Part model, mm, in its own coordinate system. A direction names the side the tool comes from. Round coordinates to 2 decimals unless told otherwise and drop trailing zeros. Write each loop counter-clockwise with the first axis right and the second up, starting at its lowest first coordinate (ties: lowest second). Pieces come first, ordered by that corner, then holes. Notation, with made-up numbers: M 1,30 L 37,30 A32 cw 37,66 Z; hole C 1.25,87 d5. An arc over 180 degrees is marked long. Use a Markdown table: item, result. Add a question column.
1) Slice it at D-D on z = 1.15. Write the cut outline in (x, y).
2) Slice it at C-C on y = 0. Write the cut outline in (x, z), plus the area to 4 significant figures.
3) Slice it at B-B on x = 0. Write the cut outline in (y, z), plus the area to 3 significant figures.
4) Wall check: probe 1 along Z at (x, y) = (1.65, -3.25); probe 2 along Y at (x, z) = (0.9, 0.3); probe 3 along Z at (x, y) = (0.15, -3.75). Give the ranges that are in metal, low to high.
5) Slice it at A-A on y = -4. Write the cut outline in (x, z), plus the area to 3 significant figures.
6) Which spindle directions (+Z, -Z, +X, -X, +Y, -Y) get a long thin tool onto all of the face, cutting with end or side? Do faces 1 (the face through (0.27, -1.22, -1.13)), 2 (the face through (0, 2.25, 1)). Say none if no direction does.
7) Drop flat-ended pins along their axis: P1, Ø0.7, axis at x = 0, y = -3, coming from the +Z side; P2, Ø2, axis at x = 0.5, z = 0.5, coming from the -Y side; P3, Ø0.7, axis at x = -1.5, y = -3.5, coming from the +Z side; P4, Ø0.7, axis at x = -1.5, y = -4, coming from the -Z side. Give the stop position or say it passes through.
```python
from build123d import *

# Parameters (mm, degrees)
SKETCH_1_W      = 4.5
SKETCH_1_H      = 4.5
EXTRUDE_1_DEPTH = 2.6
SKETCH_3_R      = 1.25
EXTRUDE_2_DEPTH = 2.3
SKETCH_4_W      = 0.6
SKETCH_4_H      = 0.2
EXTRUDE_3_DEPTH = 2.3


with BuildPart() as part:
    # 草图1 → 凸台-拉伸1 (new body)
    with BuildSketch(Plane.XY):
        Rectangle(SKETCH_1_W, SKETCH_1_H)
    extrude(amount=EXTRUDE_1_DEPTH)

    # 草图3 → 凸台-拉伸2 (add)
    with BuildSketch(Plane(origin=(0, 0, 0), x_dir=(-1, 0, 0), z_dir=(0, 0, -1))):
        Circle(SKETCH_3_R)
    extrude(amount=EXTRUDE_2_DEPTH)

    # 草图4 → 凸台-拉伸3 (add)
    with BuildSketch(Plane.XZ.offset(2.25)):
        with Locations((0, 0.1)):
            Rectangle(SKETCH_4_W, SKETCH_4_H)
        with Locations((1.5, 2.1)):
            Rectangle(SKETCH_4_W, SKETCH_4_H)
        with Locations((-1.5, 2.1)):
            Rectangle(SKETCH_4_W, SKETCH_4_H)
    extrude(amount=EXTRUDE_3_DEPTH)


solid = part.part
```
Entries:
| question | item | result |
|---|---|---|
| 1 | outline | M -2.25,-2.25 L 2.25,-2.25 L 2.25,2.25 L -2.25,2.25 Z |
| 2 | outline | M -2.25,0 L -1.25,0 L -1.25,-2.3 L 1.25,-2.3 L 1.25,0 L 2.25,0 L 2.25,2.6 L -2.25,2.6 Z |
| 2 | area | 17.45 mm^2 |
| 3 | outline | M -4.55,0 L -1.25,0 L -1.25,-2.3 L 1.25,-2.3 L 1.25,0 L 2.25,0 L 2.25,2.6 L -2.25,2.6 L -2.25,0.2 L -4.55,0.2 Z |
| 3 | area | 17.9 mm^2 |
| 4 | probe 1 | z = 2 to 2.2 |
| 4 | probe 2 | y = -2.25 to 2.25 |
| 4 | probe 3 | z = 0 to 0.2 |
| 5 | outline | M -1.8,2 L -1.2,2 L -1.2,2.2 L -1.8,2.2 Z; M -0.3,0 L 0.3,0 L 0.3,0.2 L -0.3,0.2 Z; M 1.2,2 L 1.8,2 L 1.8,2.2 L 1.2,2.2 Z |
| 5 | area | 0.360 mm^2 |
| 6 | face 1 | -Z |
| 6 | face 2 | +Z, -Z, +X, -X, +Y |
| 7 | P1 | stops at z = 0.2 |
| 7 | P2 | stops at y = -4.55 |
| 7 | P3 | stops at z = 2.2 |
| 7 | P4 | stops at z = 2 |
